Geometry check sheet. Reference: drawing and pictorial views, mm from the part's lowest x, y, z. A direction names the side the tool comes from. Round coordinates to 2 decimals unless told otherwise and drop trailing zeros. Order: outer loops, then holes, each group sorted by start corner. A loop starts at its lowest first (then second) coordinate and runs counter-clockwise, first axis right, second up.
(1) Sectioned sample at C-C, the plane x = 3. Enter the section's corners in (y, z), and give its area (3 significant figures).
(2) Depth check by flat-ended pin: pin 1 (3 mm diameter, centred on x = 7.5, z = 5, fed in from -Y); pin 2 (3.5 mm diameter, centred on y = 15, z = 3, fed in from -X). Enter the tip coordinate at first touch or a pass-through.
(3) Thickness scan on probe 1 along Y at (x, z) = (17.05, 3); probe 2 along X at (y, z) = (2.15, 3); probe 3 along X at (y, z) = (1, 2.4). Record the ranges inside material, lowest first.
(4) Sectioned sample at D-D, the plane z = 5.35. Enter the section's corners in (x, y).
(5) Tool access check on the marked faces 1 and 2. Record the directions out of +Z, -Z, +X, -X, +Y, -Y that give a thin tool (end or side, any length) a straight path to the whole face; none if there is none.
(6) Sectioned sample at A-A, the plane z = 3. Enter the section's corners in (x, y).
(7) Sectioned sample at B-B, the plane y = 7. Enter the section's corners in (x, z).
(8) Mould release check, pull along Z, two halves, no side actions. Record for the marked faces 3, 4, 5 and 6: released by +Z, released by -Z, zero draft, split by the parting line, or undercut.
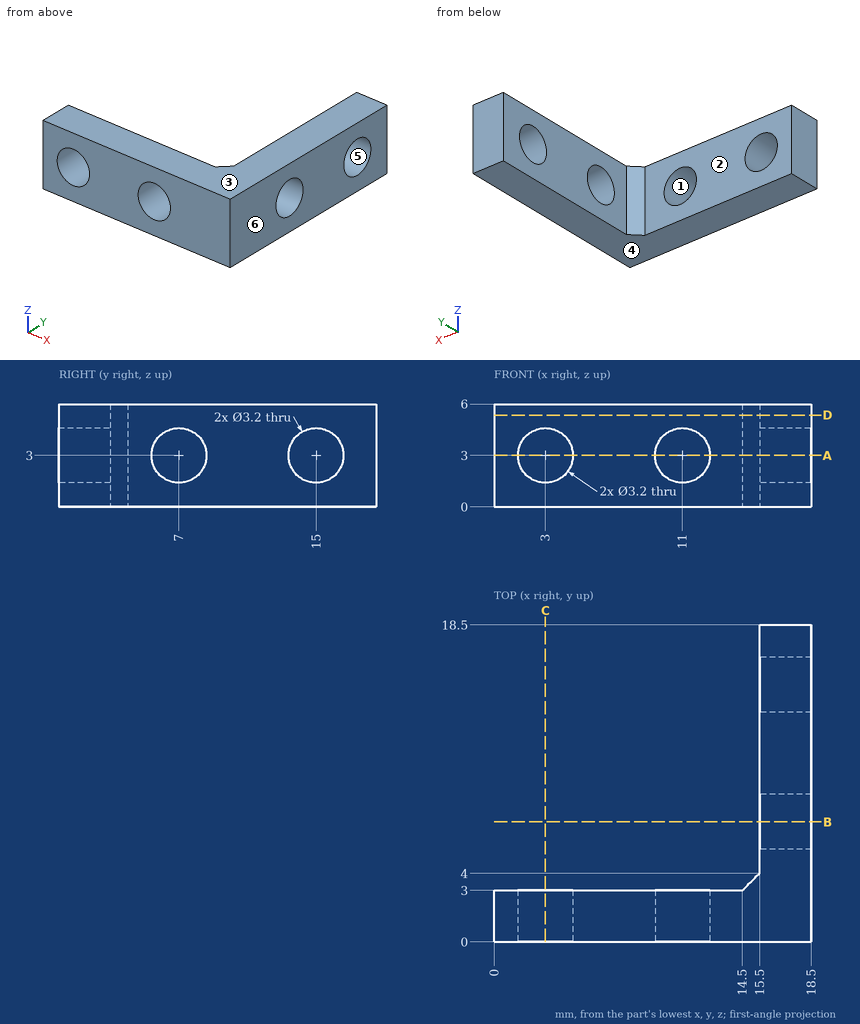
Derived:
1. outline: (0, 0) - (3, 0) - (3, 1.4) - (0, 1.4) - close; (0, 4.6) - (3, 4.6) - (3, 6) - (0, 6) - close
1. area: 8.40 mm2
2. pin 1: stops at y = 0
2. pin 2: stops at x = 15.5
3. probe 1: y = 0 to 5.4, 8.6 to 13.4, 16.6 to 18.5
3. probe 2: x = 0 to 1.4, 4.6 to 9.4, 12.6 to 18.5
3. probe 3: x = 0 to 1.52, 4.48 to 9.52, 12.48 to 18.5
4. outline: (0, 0) - (18.5, 0) - (18.5, 18.5) - (15.5, 18.5) - (15.5, 4) - (14.5, 3) - (0, 3) - close
5. face 1: +Y, -Y
5. face 2: +Z, -Z, -X, +Y
6. outline: (0, 0) - (1.4, 0) - (1.4, 3) - (0, 3) - close; (4.6, 0) - (9.4, 0) - (9.4, 3) - (4.6, 3) - close; (12.6, 0) - (18.5, 0) - (18.5, 5.4) - (15.5, 5.4) - (15.5, 4) - (14.5, 3) - (12.6, 3) - close; (15.5, 8.6) - (18.5, 8.6) - (18.5, 13.4) - (15.5, 13.4) - close; (15.5, 16.6) - (18.5, 16.6) - (18.5, 18.5) - (15.5, 18.5) - close
7. outline: (15.5, 0) - (18.5, 0) - (18.5, 1.4) - (15.5, 1.4) - close; (15.5, 4.6) - (18.5, 4.6) - (18.5, 6) - (15.5, 6) - close
8. face 3: released by +Z
8. face 4: released by -Z
8. face 5: undercut
8. face 6: zero draft
